Design review of the part built by this model. Coordinates are the model's own, in mm. Face numbers are marked on the shaded views. A direction names the side the tool comes from. Give positions to 0.01 mm unless a question says otherwise; leave off trailing zeros. Write each loop counter-clockwise with the first axis right and the second up, starting at its lowest first coordinate (ties: lowest second). Pieces come first, ordered by that corner, then holes. Notation, with made-up numbers: (21.25, -24.75) -> (70.25, -24.75) arc R27 cw to (70.25, 7.25) -> close; hole circle Ø6 at (62.5, 87). An arc over 180 degrees is marked (long way). Use CSV: the item, a comma, the result in double quotes.
```python
from build123d import *

# Parameters (mm, degrees)
F0_W     = 25.4
F0_H     = 15
F1_DEPTH = 10
F2_R     = 1.6
F3_DEPTH = 10
F5_DEPTH = 17
F7_DEPTH = 3
F8_R     = 1.2
F9_DEPTH = 3


with BuildPart() as f1:
    # F0 (on Top) → F1 (new body)
    with BuildSketch(Plane.XY):
        Rectangle(F0_W, F0_H)
    extrude(amount=F1_DEPTH)

    # F2 (on face) → F3 (cut, through all)
    with BuildSketch(Plane(origin=(0, 0, 0), x_dir=(1, 0, 0), z_dir=(0, 0, -1))):
        with Locations((-10, 5)):
            Circle(F2_R)
        with Locations((-10, -5)):
            Circle(F2_R)
        with Locations((10, -5)):
            Circle(F2_R)
        with Locations((10, 5)):
            Circle(F2_R)
    extrude(amount=-F3_DEPTH, mode=Mode.SUBTRACT)

    # F4 (on face) → F5 (join)
    with BuildSketch(Plane(origin=(0, 0, 0), x_dir=(1, 0, 0), z_dir=(0, 0, -1))):
        Polygon((-7.5, -4.5), (-7.5, -7.5), (0, -7.5), (0, 7.5), (-1.5, 7.5), (-1.5, -4.5), align=None)
        Polygon((0, 7.5), (0, -7.5), (7.5, -7.5), (7.5, -4.5), (1.5, -4.5), (1.5, 7.5), align=None)
    extrude(amount=F5_DEPTH)

    # F6 (on face) → F7 (cut, through all)
    with BuildSketch(Plane(origin=(-1.5, 0, 0), x_dir=(0, -1, 0), z_dir=(-1, 0, 0))):
        Polygon((7.5, -17), (7.5, 0), (-4.5, -17), align=None)
    extrude(amount=-F7_DEPTH, mode=Mode.SUBTRACT)

    # F8 (on face) → F9 (cut, through all)
    with BuildSketch(Plane(origin=(0, 7.5, 0), x_dir=(-1, 0, 0), z_dir=(0, 1, 0))):
        with Locations((-4.5, -14)):
            Circle(F8_R)
        with Locations((4.5, -14)):
            Circle(F8_R)
    extrude(amount=-F9_DEPTH, mode=Mode.SUBTRACT)


solid = f1.part
```
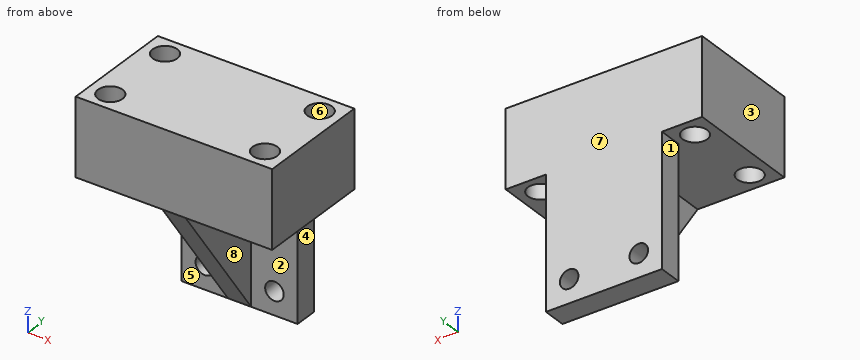
(1) Mouldability with a two-part tool opening along Y and no side actions: class the marked faces 5, 6, 7 and 8 as +Y half, -Y half, draft (parallel to the pull), parting line (faces both ways), or undercut.
Established:
face 5,"-Y half"
face 6,"undercut"
face 7,"+Y half"
face 8,"draft"
(2) Take a section at A-A (x = -4.5). Write out the cut boundary in (y, z).
Established:
outline,"(-7.5, 0) -> (4.5, 0) -> (4.5, -12.8) -> (7.5, -12.8) -> (7.5, 10) -> (-7.5, 10) -> close; (4.5, -17) -> (7.5, -17) -> (7.5, -15.2) -> (4.5, -15.2) -> close"
(3) Take a section at C-C (x = -10). Write out the cut boundary in (y, z), then the cut area to 3 significant figures.
Established:
outline,"(-7.5, 0) -> (-6.6, 0) -> (-6.6, 10) -> (-7.5, 10) -> close; (-3.4, 0) -> (3.4, 0) -> (3.4, 10) -> (-3.4, 10) -> close; (6.6, 0) -> (7.5, 0) -> (7.5, 10) -> (6.6, 10) -> close"
area,"86.0 mm2"
(4) Clearance check with flat-ended pins moving along their axes: pin 1 (1.5 mm diameter, centred on y = 6, z = -12.5, fed in from +X); pin 2 (5 mm diameter, centred on x = 5.5, z = -10, fed in from -Y); pin 3 (6 mm diameter, centred on y = 0, z = -9.5, fed in from +X). State where each tip first meets the part, or that it passes through.
Established:
pin 1,"stops at x = 7.5"
pin 2,"stops at y = 4.5"
pin 3,"stops at x = 1.5"
(5) Take a section at D-D (z = -14). Write out the cut boundary in (x, y), then the cut area to 3 significant figures.
Established:
outline,"(-7.5, 4.5) -> (-5.7, 4.5) -> (-5.7, 7.5) -> (-7.5, 7.5) -> close; (-3.3, 4.5) -> (-1.5, 4.5) -> (-1.5, 2.38) -> (1.5, 2.38) -> (1.5, 4.5) -> (3.3, 4.5) -> (3.3, 7.5) -> (-3.3, 7.5) -> close; (5.7, 4.5) -> (7.5, 4.5) -> (7.5, 7.5) -> (5.7, 7.5) -> close"
area,"37.0 mm2"
(6) Tool access review of the marked faces 1, 2, 3 and 4: name each direction out of +Z, -Z, +X, -X, +Y, -Y from which nothing blocks a thin tool from reaching the whole face with its end or side.
Established:
face 1,"-Z, -X, +Y, -Y"
face 2,"-Z, +X, -Y"
face 3,"+Z, -Z, -X, +Y, -Y"
face 4,"-Z, +X, +Y, -Y"
(7) For line 1 along X through (y, z) = (-5, 7.75); line 2 along Y through (x, z) = (10, 3.25); line 3 along Z through (x, y) = (-4.5, 5.6), list the stretches that pass through material, from the lowest coordinate up. Write a range as [from, to].
Established:
line 1,"x = [-12.7, -11.6], [-8.4, 8.4], [11.6, 12.7]"
line 2,"y = [-7.5, -6.6], [-3.4, 3.4], [6.6, 7.5]"
line 3,"z = [-17, -15.2], [-12.8, 10]"
(8) Take a section at B-B (z = 1.25). Write out the cut boundary in (x, y), then the cut area to 3 significant figures.
Established:
outline,"(-12.7, -7.5) -> (12.7, -7.5) -> (12.7, 7.5) -> (-12.7, 7.5) -> close; hole circle Ø3.2 at (-10, -5); hole circle Ø3.2 at (-10, 5); hole circle Ø3.2 at (10, -5); hole circle Ø3.2 at (10, 5)"
area,"349 mm2"
